Verification items for this drawing (mm, ordinates from the low corner). Give positions to 0.01 mm unless a question says otherwise; leave off trailing zeros. Write each loop counter-clockwise with the first axis right and the second up, starting at its lowest first coordinate (ties: lowest second). Pieces come first, ordered by that corner, then holes. Notation, with made-up numbers: (13, 82.5) -> (44, 82.5) arc R30 ccw to (44, 118.5) -> close; hole circle Ø2 at (-22, -7). An arc over 180 degrees is marked (long way). Use one line per item in the form item = value. Start each with the question number.
(1) Release check for a two-part mould opening along X. For the marked faces 1, 2 and 3 record: pulls with the +X half, pulls with the -X half, needs draft (parallel to the pull), parting line crosses it, or undercut.
(2) Depth check by flat-ended pin: pin 1 Ø8 at (x, z) = (31.5, 12) entering from +Y; pin 2 Ø6 at (x, y) = (12.5, 5.5) entering from -Z. Enter the tip coordinate at first touch or a pass-through.
(3) Section check C-C, the plane y = 7.25. Record the cut outline in (x, z), plus the area to 3 significant figures.
(4) Scan lines: L1, parallel to X at y = 4, z = 30; L2, parallel to X at y = 1.55, z = 30; L3, parallel to Z at x = 24, y = 5.5. Record each from-to range of solid material in increasing order.
(5) Section check B-B, the plane z = 30. Record the cut outline in (x, y).
(6) Section check A-A, the plane x = 30. Record the cut outline in (y, z).
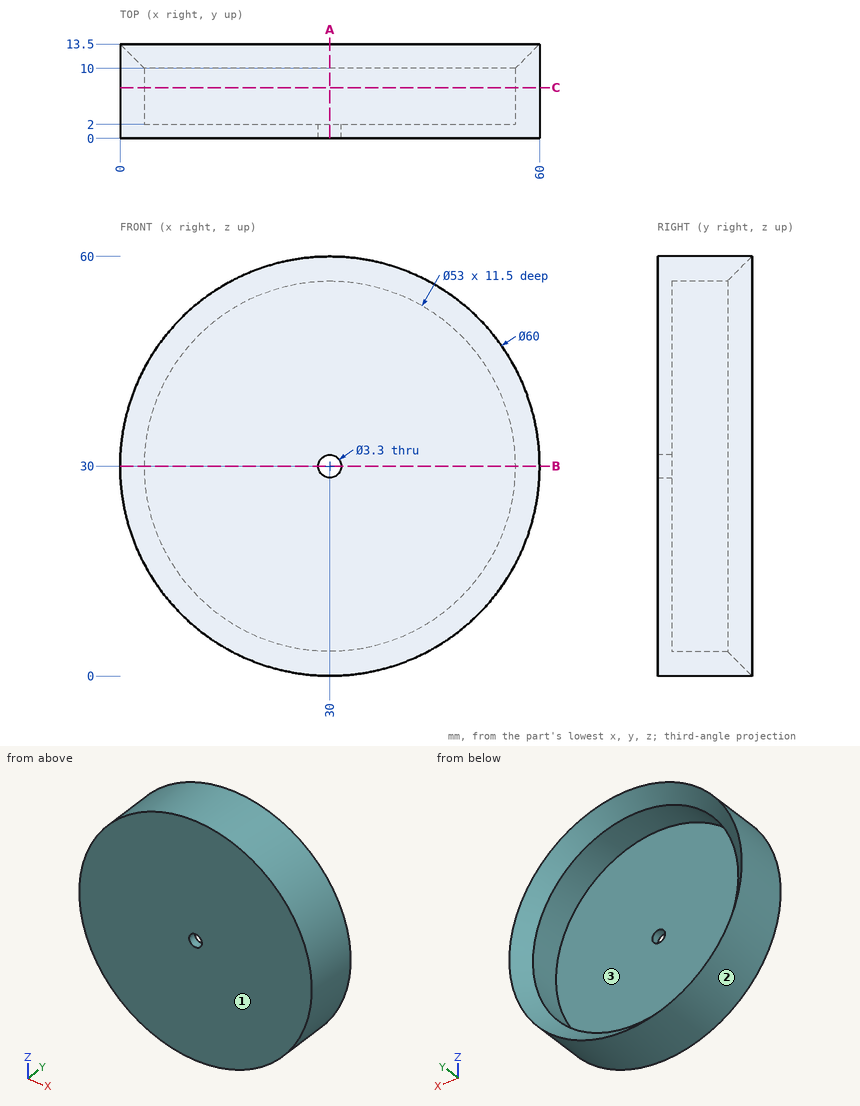
Completed:
q1.face_1 = needs draft
q1.face_2 = parting line crosses it
q1.face_3 = undercut
q2.pin_1 = 2
q2.pin_2 = 3.74
q3.outline = circle Ø60 at (30, 30); hole circle Ø53 at (30, 30)
q3.area = 621 mm²
q4.L1 = 0 to 3.5, 56.5 to 60
q4.L2 = 0 to 28.35, 31.65 to 60
q4.L3 = 0.61 to 4.19, 55.81 to 59.39
q5.outline = (0, 0) -> (28.35, 0) -> (28.35, 2) -> (3.5, 2) -> (3.5, 10) -> (0, 13.5) -> close; (31.65, 0) -> (60, 0) -> (60, 13.5) -> (56.5, 10) -> (56.5, 2) -> (31.65, 2) -> close
q6.outline = (0, 0) -> (13.5, 0) -> (10, 3.5) -> (2, 3.5) -> (2, 28.35) -> (0, 28.35) -> close; (0, 31.65) -> (2, 31.65) -> (2, 56.5) -> (10, 56.5) -> (13.5, 60) -> (0, 60) -> close
